Study the drawing (mm; zero at the part's minimum x, y, z) and answer. A direction names the side the tool comes from. Round coordinates to 2 decimals unless told otherwise and drop trailing zeros. Loops run counter-clockwise (first coordinate to the right, second up) from the corner with the lowest first, then second, coordinate; pieces in that order, holes last. Notation, with made-up numbers: M 52,-35 L 66,-35 A9 ccw 66,-21 Z; hole C 22.5,4 d5. An arc over 180 degrees is marked long. Put each result on its own line as item: value. Start each with the question number.
(1) Section A-A, the plane y = 5 is taken. Determine the outline of the cut face in (x, z), then the cut area to 3 significant figures.
(2) Flat-ended cylindrical pins translate along their axes: P1, Ø5, axis at x = 12.5, z = 2, coming from the -Y side; P2, Ø3, axis at x = 42, z = 7.5, coming from the +Y side; P3, Ø3, axis at y = 3.5, z = 4.5, coming from the -X side; P4, Ø8, axis at x = 29.5, y = 23, coming from the -Z side. Find the tip coordinate at first contact, or state that the pin passes through.
(3) Section C-C, the plane z = 7.75 is taken. Determine the outline of the cut face in (x, y), then the cut area to 3 significant figures.
(4) Section B-B, the plane x = 4 is taken. Determine the outline of the cut face in (y, z).
(5) Section D-D, the plane y = 32 is taken. Determine the outline of the cut face in (x, z), then the cut area to 3 significant figures.
(6) Which of the six approach directions +Z, -Z, +X, -X, +Y, -Y give full straight-line access (tool end or side, diameter ignored) to the marked faces 1 and 2?
(7) Straight lines are drawn through the part: line 1 (X direction, y = 9, z = 6.75); line 2 (X direction, y = 54.5, z = 5); line 3 (Y direction, x = 49.25, z = 5) (1 decimal). For each, find the intervals that lie inside material, in ascending order.
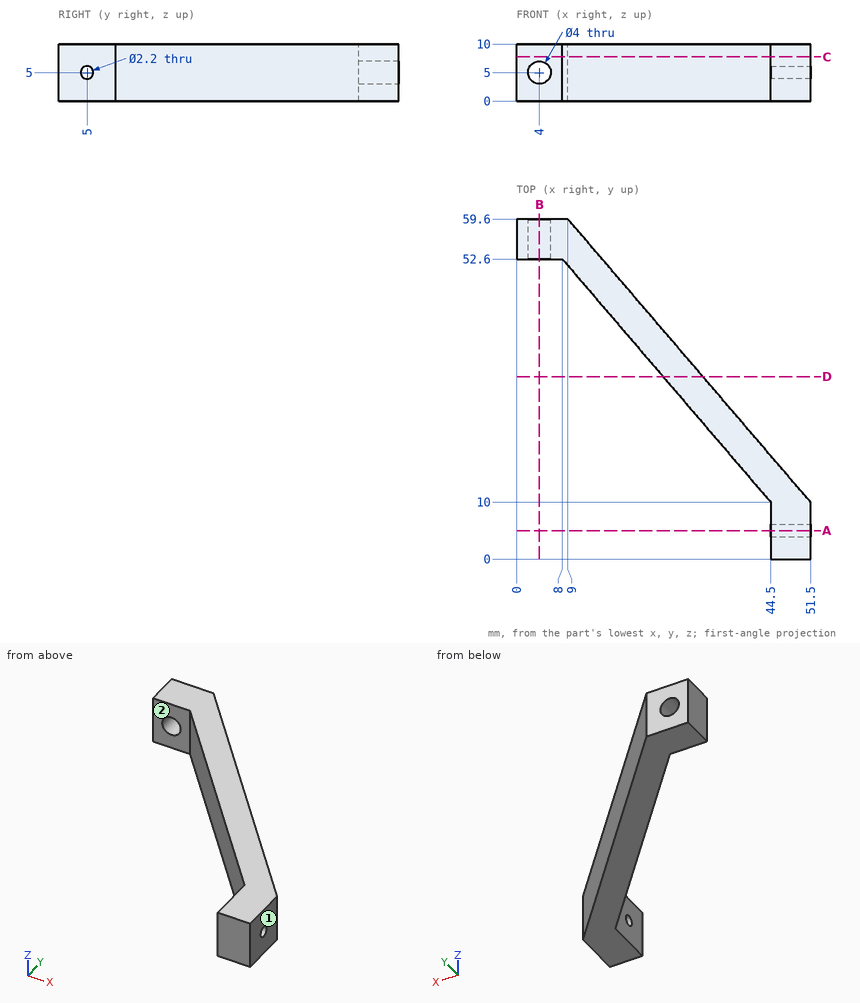
Recorded:
1. outline: M 44.5,0 L 51.5,0 L 51.5,3.9 L 44.5,3.9 Z; M 44.5,6.1 L 51.5,6.1 L 51.5,10 L 44.5,10 Z
1. area: 54.6 mm²
2. P1: stops at y = 44.43
2. P2: stops at y = 22.84
2. P3: stops at x = 44.5
2. P4: stops at z = 0
3. outline: M 0,52.6 L 8,52.6 L 44.5,10 L 44.5,0 L 51.5,0 L 51.5,10 L 9,59.6 L 0,59.6 Z
3. area: 452 mm²
4. outline: M 52.6,0 L 59.6,0 L 59.6,3 L 52.6,3 Z; M 52.6,7 L 59.6,7 L 59.6,10 L 52.6,10 Z
5. outline: M 25.65,0 L 32.65,0 L 32.65,10 L 25.65,10 Z
5. area: 70.0 mm²
6. face 1: +Z, -Z, +X, +Y, -Y
6. face 2: +Z, -Z, -X, -Y
7. line 1: x = 44.5 to 51.5
7. line 2: x = 0 to 2, 6 to 13.37
7. line 3: y = 0 to 3.9, 6.1 to 12.6
